Part model, mm, in its own coordinate system. A direction names the side the tool comes from. Coordinates: 2 decimals unless noted, no trailing zeros. Write each loop counter-clockwise with the first axis right and the second up, starting at its lowest first coordinate (ties: lowest second). Pieces come first, ordered by that corner, then holes. Notation, with made-up numbers: M 34.25,-4.5 L 50.25,-4.5 A27 ccw 50.25,16.5 Z; hole C -12.5,63 d2. An arc over 180 degrees is marked long. Use a Markdown table: item, result. Add a question column.
Q1. Slice it at D-D on x = 0. Count the separate pieces of the cut face and the enclosed holes in it, then the cut area to 3 significant figures.
Q2. Mould opens along Z. For faces 3 (the flat face through (0, 2, -0.762)), 4 (the flat face through (0.3, 3.5, 234.95)), 5 (the cylindrical face through (0.96, 3.5, 20.73)) say: released by +Z, released by -Z, zero draft, split by the parting line, or undercut.
Q3. Tool access for faces 1 (the cylindrical face through (-0.463, 3.505, 62.015)), 2 (the flat face through (0, 3.188, 116)): list every direction of +Z, -Z, +X, -X, +Y, -Y with a clear straight run to the whole face (end or side of a thin tool).
Q4. Slice it at B-B on y = 1.4. Write the cut outline in (x, z) (3 decimals), then the cut area to 3 significant figures.
Q5. Pin check, flat tips, straight feed: pin 1 Ø4 at (x, z) = (-0.01, 59.97) entering from +Y; pin 2 Ø0.9 at (x, y) = (1, 2) entering from +Z; pin 3 Ø3.5 at (x, z) = (0.5, 85) entering from -Y. Stop position of each tip, or through.
Q6. Wall check: L1, parallel to X at y = 1.9, z = 22 (3 decimals); L2, parallel to Y at x = 0.25, z = 69; L3, parallel to Z at x = 1.75, y = 1.95. Give the ranges that are in metal, low to high. Write a range as from..to.
Autodesk Inventor part; units mm, degrees
ref_plane "YZ Plane" through (0, 0, 0) normal (1, 0, 0) x (0, 1, 0)
ref_plane "XZ Plane" through (0, 0, 0) normal (0, 1, 0) x (-1, 0, 0)
ref_plane "XY Plane" through (0, 0, 0) normal (0, 0, 1) x (1, 0, 0)
sketch "Sketch1" plane through (0, 0, 0) normal (0, 0, 1) x (1, 0, 0)
  line L0 (-2.1082, 3.1877) -> (2.0912, 3.1877)
  line L1 (3.175, 2.1082) -> (3.175, 0.1305)
  line L2 (-3.1877, 0.1305) -> (-3.1877, 2.1082)
  arc A0 (-2.1082, 3.1877) -> (-3.1877, 2.1082) centre (-0.0085, 0.0085) ccw
  line L3 (-2.1082, 3.1877) -> (-3.1877, 2.1082) construction
  line L4 (-2.1082, 3.1877) -> (-0.5816, 3.1877) construction
  arc A1 (3.175, 2.1082) -> (2.0912, 3.1877) centre (-0.0009, 0.0035) ccw
  line L5 (3.8091, 0.0035) -> (3.8091, 3.5595)
  line L6 (3.5551, 3.8135) -> (-3.5569, 3.8135)
  line L7 (-3.8109, 3.5595) -> (-3.8109, 0.0035)
  arc A2 (-3.5569, 3.8135) -> (-3.8109, 3.5595) centre (-3.5569, 3.5595) ccw
  arc A3 (3.8091, 3.5595) -> (3.5551, 3.8135) centre (3.5551, 3.5595) ccw
  line L8 (-3.8109, 0.0035) -> (-3.3147, 0.0035)
  line L9 (3.302, 0.0035) -> (3.8091, 0.0035)
  arc A4 (-3.3147, 0.0035) -> (-3.1877, 0.1305) centre (-3.3147, 0.1305) ccw
  arc A5 (3.175, 0.1305) -> (3.302, 0.0035) centre (3.302, 0.1305) ccw
  point P0 (0, 0)
  point P1 (3.8091, 3.8135)
  point P2 (-3.8109, 3.8135)
  dimension "d0" = 135
  dimension "d1" = 3.81
  dimension "d2" = 3.81
  dimension "d3" = 7.62
  dimension "d4" = 3.81
  dimension "d5" = 0.254
  dimension "d6" = 0.127
extrude "Extrusion1" add sketch "Sketch1" along normal blind 234.95
sketch "Sketch2" plane through (0, 0, 0) normal (0, 0, -1) x (-1, 0, 0)
  line L0 (-3.302, 0.0035) -> (-3.8091, 0.0035)
  line L1 (3.5569, 3.8135) -> (-3.5551, 3.8135)
  line L2 (-3.8091, 3.5595) -> (-3.8091, 0.0035)
  line L3 (-3.8091, 0.0035) -> (3.8109, 0.0035)
  line L4 (3.8109, 0.0035) -> (3.8109, 3.5595)
  arc A0 (3.8109, 3.5595) -> (3.5569, 3.8135) centre (3.5569, 3.5595) ccw
  arc A1 (-3.5551, 3.8135) -> (-3.8091, 3.5595) centre (-3.5551, 3.5595) ccw
  point P0 (0, 0)
  dimension "d9" = 0.254
extrude "Extrusion2" add sketch "Sketch2" along normal blind 0.762
sketch "Sketch4" plane through (-0.0085, 3.8135, 0) normal (0, 1, 0) x (1, 0, 0)
  circle A0 centre (0.0085, -3.175) radius 2.0955
  circle A1 centre (0, -231.775) radius 2.0955
  circle A2 centre (0, -196.85) radius 2.0955
  circle A3 centre (0, -59.9694) radius 2.0955
  circle A4 centre (0, -31.5722) radius 2.0955
  circle A5 centre (0, -44.2722) radius 2.0955
  circle A6 centre (0, -18.8722) radius 2.0955
  point P0 (0.0085, 0)
  dimension "d15" = 4.191
  dimension "d16" = 4.191
  dimension "d17" = 4.191
  dimension "d18" = 4.191
  dimension "d19" = 4.191
  dimension "d20" = 4.191
  dimension "d21" = 4.191
extrude "Extrusion3" cut sketch "Sketch4" against normal blind 4.191
fillet "Fillet1" radius 0.0762 23 edges at (3.8091, 0.0035, 117.094) (-0.0009, 0.0035, -0.762) (3.7347, 3.7391, -0.762) (-0.0009, 3.8135, -0.762) (-3.7365, 3.7391, -0.762) (-3.8109, 1.7815, -0.762) (3.8091, 1.7815, -0.762) (-3.8109, 0.0035, 117.094) (-0.0063, 0.0035, 0) (3.2122, 0.0407, 234.95) (3.175, 1.1193, 234.95) (3.5556, 0.0035, 234.95) (3.7347, 3.7391, 234.95) (-0.0009, 3.8135, 234.95) (-3.7365, 3.7391, 234.95) (-3.8109, 1.7815, 234.95) (3.8091, 1.7815, 234.95) (2.6878, 2.7029, 234.95) (-0.0085, 3.1877, 234.95) (-2.7026, 2.7026, 234.95) (-3.2249, 0.0407, 234.95) (-3.5628, 0.0035, 234.95) (-3.1877, 1.1193, 234.95)
equation "\"d22\" = d20"
properties part number "hs_brace_jig" material "ABS Plastic"
Recorded:
| question | item | result |
|---|---|---|
| 1 | separate pieces | 8 |
| 1 | enclosed holes | 0 |
| 1 | area | 132 mm² |
| 2 | face 3 | released by -Z |
| 2 | face 4 | released by +Z |
| 2 | face 5 | undercut |
| 3 | face 1 | +Y, -Y |
| 3 | face 2 | +Z, -Y |
| 4 | outline | M -3.811,-0.686 A0.076 ccw -3.735,-0.762 L 3.733,-0.762 A0.076 ccw 3.809,-0.686 L 3.809,234.874 A0.076 ccw 3.733,234.95 L 3.251,234.95 A0.076 ccw 3.175,234.874 L 3.175,0 L -3.188,0 L -3.188,234.874 A0.076 ccw -3.264,234.95 L -3.735,234.95 A0.076 ccw -3.811,234.874 Z |
| 4 | area | 301 mm² |
| 5 | pin 1 | through |
| 5 | pin 2 | z = 0 |
| 5 | pin 3 | y = 3.08 |
| 6 | L1 | -3.811..-3.188, 3.175..3.809 |
| 6 | L2 | 3.19..3.81 |
| 6 | L3 | -0.76..0 |
